from build123d import *

# Parameters (mm, degrees)
F0_R     = 8
F1_DEPTH = 15
F2_DEPTH = 10


with BuildPart() as f1:
    # F0 (on Front) → F1 (new body)
    with BuildSketch(Plane.XZ):
        with BuildLine():
            Line((40, -77.8219120814), (40, 77.8219120814))
            ThreePointArc((40, 77.8219120814), (0, 87.5), (-40, 77.8219120814))
            Line((-40, 77.8219120814), (-40, -77.8219120814))
            ThreePointArc((-40, -77.8219120814), (0, -87.5), (40, -77.8219120814))
        make_face()
        Circle(F0_R, mode=Mode.SUBTRACT)
    extrude(amount=F1_DEPTH)

    # F0 (on Front) → F2 (join)
    with BuildSketch(Plane.XZ):
        with BuildLine():
            ThreePointArc((-40, 77.8219120814), (0, 87.5), (40, 77.8219120814))
            Line((40, 77.8219120814), (40, 88.9170962189))
            ThreePointArc((40, 88.9170962189), (0, 97.5), (-40, 88.9170962189))
            Line((-40, 88.9170962189), (-40, 77.8219120814))
        make_face()
        with BuildLine():
            Line((40, -88.9170962189), (40, -77.8219120814))
            ThreePointArc((40, -77.8219120814), (0, -87.5), (-40, -77.8219120814))
            Line((-40, -77.8219120814), (-40, -88.9170962189))
            ThreePointArc((-40, -88.9170962189), (0, -97.5), (40, -88.9170962189))
        make_face()
    extrude(amount=F2_DEPTH)


solid = f1.part
Geometry check sheet. Reference: the model listing, model coordinates, mm. A direction names the side the tool comes from. Round coordinates to 2 decimals unless told otherwise and drop trailing zeros. Order: outer loops, then holes, each group sorted by start corner. A loop starts at its lowest first (then second) coordinate and runs counter-clockwise, first axis right, second up. Notation, with made-up numbers: M -12,-26.5 L 15,-26.5 A7 cw 15,-17.5 Z; hole C -28,-13 d5. An arc over 180 degrees is marked long. Answer in a Markdown table with one row per item. Add a question column.
Item 1: Sectioned sample at B-B, the plane z = 0. Enter the section's corners in (x, y).
Item 2: Draft check along Z on faces 4 (the face through (0.6, -4.9, 97.5)), 5 (the face through (-0.6, -4.9, -97.5)), 6 (the face through (-40, -7, 1)), 7 (the face through (-1.73, -7.4, -7.81)). Enter one of: released by +Z, released by -Z, zero draft, split by the parting line, or undercut.
Item 3: Set-up check for faces 1 (the face through (8.3, -15, 1.2)), 2 (the face through (-0.58, -12.46, -87.5)), 3 (the face through (0.58, -12.46, 87.5)): record each of +Z, -Z, +X, -X, +Y, -Y from which the full face is reachable in a straight line by a thin tool's end or side.
Item 4: Sectioned sample at A-A, the plane x = 0. Enter the section's corners in (y, z).
Item 5: Depth check by flat-ended pin: pin 1 Ø2 at (x, y) = (21.5, -3) entering from +Z; pin 2 Ø9.5 at (x, z) = (0, 0) entering from -Y; pin 3 Ø3 at (x, y) = (-6, -13) entering from -Z; pin 4 Ø3 at (x, y) = (14.5, -10.5) entering from -Z. Enter the tip coordinate at first touch or a pass-through.
Item 6: Sectioned sample at D-D, the plane x = -12. Enter the section's corners in (y, z).
Item 7: Sectioned sample at C-C, the plane y = -5.5. Enter the section's corners in (x, z), plus the area to 3 significant figures.
Item 8: Material ranges on L1, parallel to Z at x = 0, y = -4.5; L2, parallel to Y at x = -27, z = 89; L3, parallel to Z at x = -1, y = -11.5, recorded low to high. Write a range as [from, to].
Filled in:
| question | item | result |
|---|---|---|
| 1 | outline | M -40,-15 L -8,-15 L -8,0 L -40,0 Z; M 8,-15 L 40,-15 L 40,0 L 8,0 Z |
| 2 | face 4 | released by +Z |
| 2 | face 5 | released by -Z |
| 2 | face 6 | zero draft |
| 2 | face 7 | undercut |
| 3 | face 1 | +Z, -Z, +X, -X, -Y |
| 3 | face 2 | -Z, -Y |
| 3 | face 3 | +Z, -Y |
| 4 | outline | M -15,-87.5 L -10,-87.5 L -10,-97.5 L 0,-97.5 L 0,-8 L -15,-8 Z; M -15,8 L 0,8 L 0,97.5 L -10,97.5 L -10,87.5 L -15,87.5 Z |
| 5 | pin 1 | stops at z = 95.32 |
| 5 | pin 2 | passes through |
| 5 | pin 3 | stops at z = -87.38 |
| 5 | pin 4 | stops at z = -96.62 |
| 6 | outline | M -15,-86.67 L -10,-86.67 L -10,-96.76 L 0,-96.76 L 0,96.76 L -10,96.76 L -10,86.67 L -15,86.67 Z |
| 7 | outline | M -40,-88.92 A97.5 ccw 40,-88.92 L 40,88.92 A97.5 ccw -40,88.92 Z; hole C 0,0 d16 |
| 7 | area | 14,900 mm² |
| 8 | L1 | z = [-97.5, -8], [8, 97.5] |
| 8 | L2 | y = [-10, 0] |
| 8 | L3 | z = [-87.49, -7.94], [7.94, 87.49] |
